The model under review builds one solid part; all positions refer to its coordinate system, in mm. A direction names the side the tool comes from. Coordinates: 2 decimals unless noted, no trailing zeros. Loops run counter-clockwise (first coordinate to the right, second up) from the corner with the lowest first, then second, coordinate; pieces in that order, holes last. Notation, with made-up numbers: M 89.25,86.25 L 141.25,86.25 A21 cw 141.25,100.25 Z; hole C 54,12.5 d8. An arc over 180 degrees is marked long. Use one line per item in the form item = value.
```python
from build123d import *

# Parameters (mm, degrees)
BOSS_EXTRUDE1_DEPTH = 52
BOSS_EXTRUDE2_DEPTH = 1
BOSS_EXTRUDE3_START = -52
BOSS_EXTRUDE3_DEPTH = 1
SKETCH4_W           = 18.000000053
SKETCH4_H           = 12.9
SKETCH4_W_2         = 18
CUT_EXTRUDE1_DEPTH  = 2
SKETCH5_R           = 3.3
SKETCH5_R_2         = 2.25
BOSS_EXTRUDE4_DEPTH = 22


with BuildPart() as part:
    # Sketch2 → Boss-Extrude1 (new body)
    with BuildSketch(Plane.XY):
        Polygon((-21.624010924, -70.352088598), (-7.5, -25.4), (-27.5, -25.4), (-25.794353309, -62.332940574), (-23.792221644, -62.332940574), (-25.405503813, -27.4), (-10.224802214, -27.4), (-23.085991045, -68.332940574), (-23.515128079, -68.332940574), (-25.517259745, -68.332940574), (-25.424010924, -70.352088598), align=None)
    extrude(amount=-BOSS_EXTRUDE1_DEPTH)

    # Sketch2<3> → Boss-Extrude2 (add)
    with BuildSketch(Plane.XY):
        Polygon((-23.515128079, -68.332940574), (-23.085991045, -68.332940574), (-10.224802214, -27.4), (-25.405503813, -27.4), align=None)
    extrude(amount=-BOSS_EXTRUDE2_DEPTH)

    # Sketch2<4> → Boss-Extrude3 (add)
    with BuildSketch(Plane.XY.offset(BOSS_EXTRUDE3_START)):
        Polygon((-23.515128079, -68.332940574), (-23.085991045, -68.332940574), (-10.224802214, -27.4), (-25.405503813, -27.4), align=None)
    extrude(amount=BOSS_EXTRUDE3_DEPTH)

    # Sketch4 → Cut-Extrude1 (cut)
    with BuildSketch(Plane.XZ.offset(25.4)):
        with Locations((-17.500000027, -7.65)):
            Rectangle(SKETCH4_W, SKETCH4_H)
        with Locations((-17.5, -44.65)):
            Rectangle(SKETCH4_W_2, SKETCH4_H)
    extrude(amount=CUT_EXTRUDE1_DEPTH, mode=Mode.SUBTRACT)

    # Sketch5 → Boss-Extrude4 (add)
    with BuildSketch(Plane(origin=(0, 0, -15), x_dir=(-1, 0, 0), z_dir=(0, 0, -1))):
        with BuildLine():
            Line((7.5, -22.955849111), (7.5, -25.4))
            Line((7.5, -25.4), (27.5, -25.4))
            Line((27.5, -25.4), (27.5, 0.016796875))
            ThreePointArc((27.5, 0.016796875), (26.360398691, 7.577422908), (23.04284729, 14.466226133))
            ThreePointArc((23.04284729, 14.466226133), (22.876796583, 15.153555184), (23.20688118, 15.778885673))
            Line((23.20688118, 15.778885673), (25.185252728, 17.527214018))
            ThreePointArc((25.185252728, 17.527214018), (20.527214018, 17.814747272), (20.814747272, 22.472785982))
            Line((20.814747272, 22.472785982), (18.598905377, 20.514600122))
            ThreePointArc((18.598905377, 20.514600122), (17.974550182, 20.264645495), (17.333078903, 20.466663618))
            Line((17.333078903, 20.466663618), (15.787974775, 15.080867994))
            ThreePointArc((15.787974775, 15.080867994), (20.592977306, -4.399589042), (7.5, -19.60321364))
            Line((7.5, -19.60321364), (7.5, -22.955849111))
        make_face()
        with Locations((23, 20)):
            Circle(SKETCH5_R)
        with Locations((23, 20)):
            Circle(SKETCH5_R_2, mode=Mode.SUBTRACT)
    extrude(amount=BOSS_EXTRUDE4_DEPTH)


solid = part.part
```
1. The part is to be moulded in two halves that separate along X. For faces 5 (the face through (-18, -26, -14.1)), 6 (the face through (-26.392, 7.475, -25.846)), 7 (the face through (-24, -68.333, -26)), say which applies: pulls with the +X half, pulls with the -X half, needs draft (parallel to the pull), parting line crosses it, or undercut.
Response values:
face_5 = undercut
face_6 = pulls with the -X half
face_7 = needs draft
2. Insertion check: P1, Ø0.6, axis at y = -26, z = -8, coming from the -X side; P2, Ø10, axis at x = -24.5, y = -17.5, coming from the -Z side; P3, Ø5, axis at x = -23, y = 20, coming from the +Z side; P4, Ø1.5, axis at y = 3.5, z = -13.5, coming from the +X side. Each pin has a flat end and moves straight along its axis. Give the tip position at first contact, or say it passes through.
Response values:
P1 = -27.49
P2 = -37
P3 = -15
P4 = through
3. Add section B-B (z = -34.5). State the section outline as (x, y) points, then the cut area to 3 significant figures.
Response values:
outline = M -27.5,-25.4 L -25.79,-62.33 L -23.79,-62.33 L -25.41,-27.4 L -10.22,-27.4 L -23.09,-68.33 L -25.52,-68.33 L -25.42,-70.35 L -21.62,-70.35 L -7.5,-25.4 L -7.5,-19.6 A21.88 cw -15.79,15.08 L -17.33,20.47 A1 cw -18.6,20.51 L -20.81,22.47 A3.3 ccw -25.19,17.53 L -23.21,15.78 A1 cw -23.04,14.47 A25.65 ccw -27.5,0.02 Z; hole C -23,20 d4.5
area = 660 mm^2
4. Add section D-D (y = -24.5). State the section outline as (x, z) points, then the cut area to 3 significant figures.
Response values:
outline = M -27.5,-37 L -7.5,-37 L -7.5,-15 L -27.5,-15 Z
area = 440 mm^2
5. Add section C-C (y = -56). State the section outline as (x, z) points, then the cut area to 3 significant figures.
Response values:
outline = M -26.09,-52 L -17.11,-52 L -17.11,0 L -26.09,0 Z; hole M -24.08,-51 L -19.21,-51 L -19.21,-1 L -24.08,-1 Z
area = 223 mm^2
6. Machinability: for faces 1 (the face through (-22, -6, -37)), 2 (the face through (-10, -27.4, -45)), 3 (the face through (-24.588, -45.111, -25.65)), 4 (the face through (-24.18, 16.64, -25.85)), which of the approach directions +Z, -Z, +X, -X, +Y, -Y give a long, thin tool a straight path to every point of the face, cutting with its end or side? Answer none if there is none.
Response values:
face_1 = -Z, +X, -X, +Y
face_2 = +Y
face_3 = none
face_4 = +Z, -Z, -X
7. Wall thickness on line 1 along Z through (x, y) = (-18.5, -26); line 2 along Z through (x, y) = (-24.5, -39.5); line 3 along X through (y, z) = (-29.5, -21): over which ranges is each line inside the solid? List them lowest first. Write a range as from..to.
Response values:
line_1 = -52..-51.1, -38.2..-14.1, -1.2..0
line_2 = -52..-51, -1..0
line_3 = -27.31..-25.31, -10.88..-8.79
8. Add section A-A (z = -43.5). State the section outline as (x, y) points.
Response values:
outline = M -27.5,-25.4 L -25.79,-62.33 L -23.79,-62.33 L -25.41,-27.4 L -26.5,-27.4 L -26.5,-25.4 Z; M -25.52,-68.33 L -25.42,-70.35 L -21.62,-70.35 L -7.5,-25.4 L -8.5,-25.4 L -8.5,-27.4 L -10.22,-27.4 L -23.09,-68.33 Z
